Design review of the part built by this model. Coordinates are the model's own, in mm. A direction names the side the tool comes from. Give positions to 0.01 mm unless a question says otherwise; leave off trailing zeros. Write each loop counter-clockwise with the first axis right and the second up, starting at its lowest first coordinate (ties: lowest second). Pieces come first, ordered by that corner, then holes. Notation, with made-up numbers: M 51,79.5 L 76,79.5 A37 ccw 76,117.5 Z; hole C 1.25,41.5 d2. An arc over 180 degrees is marked long. One line per item, written item: value. Start each with the question number.
```python
from build123d import *

# Parameters (mm, degrees)
F0_R     = 9.525
F0_R_2   = 0.4445
F1_DEPTH = 2.54
F2_R     = 1.778
F3_DEPTH = 1.27
F4_R     = 9.525
F4_R_2   = 5.4
F5_DEPTH = 46


# Not quite as in the source:
# - a feature names something its author has since deleted; it is built from what else it names


with BuildPart() as f1:
    # F0 (on Top) → F1 (new body)
    with BuildSketch(Plane.XY):
        Circle(F0_R)
        with Locations((0, -3.0520705041)):
            Circle(F0_R_2, mode=Mode.SUBTRACT)
        with Locations((0, 5.08)):
            Circle(F0_R_2, mode=Mode.SUBTRACT)
    extrude(amount=F1_DEPTH)

    # F2 (on face) → F3 (cut)
    with BuildSketch(Plane.XY.offset(2.54)):
        Circle(F2_R)
        with BuildLine():
            ThreePointArc((9.525, 0), (9.4846037847, 0.876308192), (9.3637577853, 1.7451834108))
            ThreePointArc((9.3637577853, 1.7451834108), (7.7122697392, -0.0678733407), (9.3315921315, -1.9097155001))
            ThreePointArc((9.3315921315, -1.9097155001), (9.4765246808, -0.9597421392), (9.525, 0))
        make_face()
        with BuildLine():
            ThreePointArc((-1.7451834108, 9.3637577853), (0.0678733407, 7.7122697392), (1.9097155001, 9.3315921315))
            ThreePointArc((1.9097155001, 9.3315921315), (0.0838233823, 9.5246311551), (-1.7451834108, 9.3637577853))
        make_face()
        with BuildLine():
            ThreePointArc((-1.9097155001, -9.3315921315), (-0.0838233823, -9.5246311551), (1.7451834108, -9.3637577853))
            ThreePointArc((1.7451834108, -9.3637577853), (-0.0678733407, -7.7122697392), (-1.9097155001, -9.3315921315))
        make_face()
        with BuildLine():
            ThreePointArc((-9.3637577853, -1.7451834108), (-7.7122697392, 0.0678733407), (-9.3315921315, 1.9097155001))
            ThreePointArc((-9.3315921315, 1.9097155001), (-9.5246311551, 0.0838233823), (-9.3637577853, -1.7451834108))
        make_face()
    extrude(amount=-F3_DEPTH, mode=Mode.SUBTRACT)

    # F4 (on face) → F5 (join)
    with BuildSketch(Plane(origin=(0, 0, 0), x_dir=(1, 0, 0), z_dir=(0, 0, -1))):
        Circle(F4_R)
        with BuildLine():
            ThreePointArc((5.0657137645, 6.9156561732), (7.6457042676, 3.8769785274), (8.5725, 0))
            ThreePointArc((8.5725, 0), (-3.8769785274, -7.6457042676), (-5.0657137645, 6.9156561732))
            ThreePointArc((-5.0657137645, 6.9156561732), (0, 9.4230005905), (5.0657137645, 6.9156561732))
        make_face(mode=Mode.SUBTRACT)
        with BuildLine():
            ThreePointArc((6.3709300865, 3.0520705041), (6.0358122236, 5.0911195392), (5.0657137645, 6.9156561732))
            ThreePointArc((5.0657137645, 6.9156561732), (0, 8.5725), (-5.0657137645, 6.9156561732))
            ThreePointArc((-5.0657137645, 6.9156561732), (-2.0390490351, -2.9837417196), (6.3709300865, 3.0520705041))
        make_face()
        with Locations((0, 3.0520705041)):
            Circle(F4_R_2, mode=Mode.SUBTRACT)
        with BuildLine():
            ThreePointArc((-5.0657137645, 6.9156561732), (0, 8.5725), (5.0657137645, 6.9156561732))
            ThreePointArc((5.0657137645, 6.9156561732), (0, 9.4230005905), (-5.0657137645, 6.9156561732))
        make_face()
    extrude(amount=F5_DEPTH)


solid = f1.part
```
Q1. Take a section at C-C, the plane z = -21.5. State how many separate pieces and enclosed holes the cut face has, then the cut area to 3 significant figures.
Q2. Take a section at A-A, the plane x = 0. Give the boundary of the cut face in (y, z) (1 decimal), then the cut area to 3 significant figures.
Q3. Wall thickness on line 1 (Y direction, x = 0, z = 2); line 2 (Y direction, x = 0, z = -15.5) (1 decimal); line 3 (Y direction, x = 1.5, z = -18.5): over which ranges is each line inside the solid? List them lowest first. Write a range as from..to.
Q4. Machinability: for faces 4 (the face through (-7.713, 0.03, 1.914)), 5 (the face through (0, 0, 1.27)), 6 (the face through (-0.03, -7.713, 1.914)), which of the approach directions +Z, -Z, +X, -X, +Y, -Y give a long, thin tool a straight path to every point of the face, cutting with its end or side? Answer none if there is none.
Q5. The part is to be moulded in two halves that separate along Y. For faces 1 (the face through (0, -9, 1.27)), 2 (the face through (7.713, -0.03, 1.914)), 3 (the face through (0.03, 7.713, 1.914)), say which applies: pulls with the +Y half, pulls with the -Y half, needs draft (parallel to the pull), parting line crosses it, or undercut.
Q6. Take a section at D-D, the plane x = -7.25. Give the boundary of the cut face in (y, z), then the cut area to 3 significant figures.
Q7. For P1, Ø4, axis at x = -0.5, y = -0.5, coming from the +Z side; P2, Ø0.5, axis at x = 9, y = -1, coming from the +Z side; P3, Ø1, axis at x = -1.5, y = -2.5, coming from the -Z side; P4, Ø2, axis at y = 7.5, z = -31, coming from the -X side, all flat-tipped, find the tip position at first contact; note any pin that passes through.
Q8. Take a section at B-B, the plane y = 5.08. Give the boundary of the cut face in (x, z).
Results list:
1. separate pieces: 1
1. enclosed holes: 2
1. area: 83.7 mm^2
2. outline: M -9.5,-46 L -8.5,-46 L -8.5,0 L -3.5,0 L -3.5,2.5 L -7.7,2.5 L -7.7,1.3 L -9.5,1.3 Z; M -2.6,0 L 2.3,0 L 2.3,-46 L 3.3,-46 L 3.3,0 L 4.6,0 L 4.6,2.5 L 1.8,2.5 L 1.8,1.3 L -1.8,1.3 L -1.8,2.5 L -2.6,2.5 Z; M 5.5,0 L 8.6,0 L 8.6,-46 L 9.5,-46 L 9.5,1.3 L 7.7,1.3 L 7.7,2.5 L 5.5,2.5 Z
2. area: 173 mm^2
3. line 1: y = -7.71..-3.5, -2.61..-1.78, 1.78..4.64, 5.52..7.71
3. line 2: y = -9.5..-8.5, 2.3..3.3, 8.6..9.5
3. line 3: y = -9.41..-8.24, 2.14..3.14, 8.44..9.41
4. face 4: +Z, -X
4. face 5: +Z
4. face 6: +Z, -Y
5. face 1: needs draft
5. face 2: undercut
5. face 3: pulls with the +Y half
6. outline: M -6.18,-46 L -4.57,-46 L -4.57,0 L 4.57,0 L 4.57,-46 L 6.18,-46 L 6.18,2.54 L -6.18,2.54 Z
6. area: 179 mm^2
7. P1: stops at z = 2.54
7. P2: stops at z = 1.27
7. P3: stops at z = 0
7. P4: stops at x = -6.96
8. outline: M -8.06,-46 L -6.91,-46 L -6.91,0 L -0.44,0 L -0.44,2.54 L -8.06,2.54 Z; M 0.44,0 L 6.91,0 L 6.91,-46 L 8.06,-46 L 8.06,2.54 L 0.44,2.54 Z
